For this review, take the finished solid that the model builds, in its own axes (mm). A direction names the side the tool comes from. Coordinates: 2 decimals unless noted, no trailing zeros. Order: outer loops, then holes, each group sorted by start corner. A loop starts at its lowest first (then second) coordinate and runs counter-clockwise, first axis right, second up.
from build123d import *

# Parameters (mm, degrees)
FILLET1_R          = 0.75
SKETCH2_R          = 8.73
CUT_EXTRUDE1_DEPTH = 5


with BuildPart() as part:
    # Sketch1 → Revolve1 (revolve)
    with BuildSketch(Plane.XY, mode=Mode.PRIVATE) as revolve1_sk:
        Polygon((-3.57, 50), (-3.57, 0), (0, 0), (0, 45), align=None)
        Polygon((0, 45), (0, 0), (3.57, 0), (3.57, 50), align=None)
    revolve(revolve1_sk.sketch.rotate(Axis((0, 0, 0), (1, 0, 0)), 90), axis=Axis((0, 0, 0), (1, 0, 0)))

    # Fillet1
    fillet1_edges = [part.edges().sort_by_distance(p)[0] for p in [
        (-3.57, 0, -50),
        (3.57, 0, -50),
    ]]
    fillet(fillet1_edges, radius=FILLET1_R)

    # Sketch2 → Cut-Extrude1 (cut, symmetric)
    with BuildSketch(Plane(origin=(0, 0, 0), x_dir=(0, 0, -1), z_dir=(1, 0, 0))):
        with Locations(Location((0, 0, 0), (0, 0, 180))):
            Circle(SKETCH2_R)
    extrude(amount=CUT_EXTRUDE1_DEPTH, both=True, mode=Mode.SUBTRACT)


solid = part.part
1. To check wall thickness, follow L1, parallel to Z at x = -2.5, y = -4.5; L2, parallel to Y at x = -1, z = -4.5; L3, parallel to X at y = -23, z = -40. State the ranges of each line that lie inside material, in increasing order.
Answer below:
L1: z = -48.13 to -7.48, 7.48 to 48.13
L2: y = -46.18 to -7.48, 7.48 to 46.18
L3: x = -3.57 to -0.81, 0.81 to 3.57
2. The part is to be moulded in two halves that separate along X. For faces 3 (the face through (3.57, 10, 1)), 4 (the face through (-0.14, -13.57, 43.11)), 5 (the face through (0.05, -8.656, -1.136)), say which applies: +X half, -X half, draft (parallel to the pull), parting line (faces both ways), or undercut.
Answer below:
face 3: +X half
face 4: undercut
face 5: draft
3. Clearance check with flat-ended pins moving along their axes: pin 1 Ø3 at (x, y) = (-2.5, -10.5) entering from +Z; pin 2 Ø4 at (x, y) = (-2.5, -24) entering from +Z; pin 3 Ø2 at (x, z) = (1, -29) entering from -Y. State where each tip first meets the part, or that it passes through.
Answer below:
pin 1: stops at z = 47.56
pin 2: stops at z = 43.11
pin 3: stops at y = -38.16
4. Machinability: for faces 1 (the face through (-3.57, 10, -1)), 2 (the face through (0.1, 27.5, -35.8)), which of the approach directions +Z, -Z, +X, -X, +Y, -Y give a long, thin tool a straight path to every point of the face, cutting with its end or side? Answer none if there is none.
Answer below:
face 1: +Z, -Z, -X, +Y, -Y
face 2: none
5. Take a section at A-A, the plane y = 0. Give the boundary of the cut face in (x, z).
Answer below:
outline: (-3.57, -47.66) arc R0.75 ccw to (-2.21, -48.09) - (0, -45) - (2.21, -48.09) arc R0.75 ccw to (3.57, -47.66) - (3.57, -8.73) - (-3.57, -8.73) - close; (-3.57, 8.73) - (3.57, 8.73) - (3.57, 47.66) arc R0.75 ccw to (2.21, 48.09) - (0, 45) - (-2.21, 48.09) arc R0.75 ccw to (-3.57, 47.66) - close
